```python
from build123d import *

# Parameters (mm, degrees)
SKETCH_1_RX              = 300
SKETCH_1_RY              = 300
SKETCH_1_R               = 50
EXTRUDE_1_DEPTH          = 60
CUT_EXTRUDE_1_DEPTH      = 429.485705713
CUT_EXTRUDE_1_DEPTH_BACK = 429.485705713
CUT_EXTRUDE_2_DEPTH      = 429.485705867
CUT_EXTRUDE_2_DEPTH_BACK = 429.485705867
SKETCH_4_W               = 200
SKETCH_4_H               = 100
CUT_EXTRUDE_3_DEPTH      = 429.485705867


with BuildPart() as part:
    # 草图1 → 凸台-拉伸1 (new body)
    with BuildSketch(Plane(origin=(0, 0, 0), x_dir=(1, 0, 0), z_dir=(0, 1, 0))):
        with Locations((0, 0)):
            Ellipse(SKETCH_1_RX, SKETCH_1_RY)
        with Locations(Location((0, 0, 0), (0, 0, 270))):
            Circle(SKETCH_1_R, mode=Mode.SUBTRACT)
    extrude(amount=EXTRUDE_1_DEPTH)

    # 草图2 → 切除-拉伸1 (cut, two sides: drawn at the far end of the back side and taken through both)
    with BuildSketch(Plane.XY.offset(-CUT_EXTRUDE_1_DEPTH_BACK)):
        with BuildLine():
            ThreePointArc((0, 38), (-8, 30), (0, 22))
            Line((0, 22), (0, 38))
        make_face()
        with BuildLine():
            Line((0, 38), (0, 22))
            ThreePointArc((0, 22), (5.656854249, 24.343145751), (8, 30))
            ThreePointArc((8, 30), (5.656854249, 35.656854249), (0, 38))
        make_face()
        with BuildLine():
            ThreePointArc((0, 38), (-8, 30), (0, 22))
            Line((0, 22), (0, 38))
        make_face()
        with BuildLine():
            Line((0, 38), (0, 22))
            ThreePointArc((0, 22), (5.656854249, 24.343145751), (8, 30))
            ThreePointArc((8, 30), (5.656854249, 35.656854249), (0, 38))
        make_face()
    extrude(amount=CUT_EXTRUDE_1_DEPTH + CUT_EXTRUDE_1_DEPTH_BACK, mode=Mode.SUBTRACT)

    # 草图3 → 切除-拉伸2 (cut, two sides: drawn at the far end of the back side and taken through both)
    with BuildSketch(Plane(origin=(0, 0, 0), x_dir=(0, 0, -1), z_dir=(1, 0, 0)).offset(-CUT_EXTRUDE_2_DEPTH_BACK)):
        with BuildLine():
            ThreePointArc((0, 38), (-8, 30), (0, 22))
            Line((0, 22), (0, 38))
        make_face()
        with BuildLine():
            Line((0, 38), (0, 22))
            ThreePointArc((0, 22), (5.656854249, 24.343145751), (8, 30))
            ThreePointArc((8, 30), (5.656854249, 35.656854249), (0, 38))
        make_face()
        with BuildLine():
            ThreePointArc((0, 38), (-8, 30), (0, 22))
            Line((0, 22), (0, 38))
        make_face()
        with BuildLine():
            Line((0, 38), (0, 22))
            ThreePointArc((0, 22), (5.656854249, 24.343145751), (8, 30))
            ThreePointArc((8, 30), (5.656854249, 35.656854249), (0, 38))
        make_face()
    extrude(amount=CUT_EXTRUDE_2_DEPTH + CUT_EXTRUDE_2_DEPTH_BACK, mode=Mode.SUBTRACT)

    # 草图4 → 切除-拉伸3 (cut, through all)
    with BuildSketch(Plane(origin=(0, 60, 0), x_dir=(1, 0, 0), z_dir=(0, 1, 0))):
        Rectangle(SKETCH_4_W, SKETCH_4_H)
    extrude(amount=-CUT_EXTRUDE_3_DEPTH, mode=Mode.SUBTRACT)


solid = part.part
```
Geometry: final body of the model. Coordinates: model frame, mm. A direction names the side the tool comes from. Coordinates: 2 decimals unless noted, no trailing zeros. Answer as CSV lines item,"result".
Q1. Set-up query: faces 1 (the flat face through (-4, 60, 62)), 2 (the flat face through (100, 30, 12)). Return all of +Z, -Z, +X, -X, +Y, -Y with unobstructed straight access to the full face (end or side cutting, diameter ignored); none if empty.
Answers:
face 1,"+Z, -Z, +X, -X, +Y"
face 2,"+Y, -Y"
Q2. Line query: probe 1 along Z at (x, y) = (-98, 17.5); probe 2 along X at (y, z) = (6, -38.5); probe 3 along X at (y, z) = (25, 24.5). Output: solid intervals per line, ascending. Write a range as [from, to].
Answers:
probe 1,"z = [-283.54, -50], [50, 283.54]"
probe 2,"x = [-297.52, -100], [100, 297.52]"
probe 3,"x = [-299, -100], [100, 299]"
Q3. First-contact query: P1, Ø10, axis at x = 134, y = 44.5, coming from the -Z side; P2, Ø5, axis at y = 44.5, z = -25.5, coming from the +X side; P3, Ø1, axis at x = 156, y = 39.5, coming from the +Z side. Flat tips, straight axial feed; report the tip coordinate or a pass-through.
Answers:
P1,"stops at z = -270.85"
P2,"stops at x = 299.12"
P3,"stops at z = 256.55"
Q4. Draft query along Z for faces 3 (the flat face through (-1, 44, -50)), 4 (the flat face through (-100, 30, 12)), 5 (the flat face through (-4, 0, 62)). Return one class per face: pulls with the +Z half, pulls with the -Z half, needs draft (parallel to the pull), parting line crosses it, or undercut.
Answers:
face 3,"undercut"
face 4,"undercut"
face 5,"needs draft"
